The listing builds one solid part. Answer for the finished solid, in the listing's coordinates (mm). Face numbers are marked on the shaded views. A direction names the side the tool comes from. Coordinates: 2 decimals unless noted, no trailing zeros. Order: outer loops, then holes, each group sorted by start corner. A loop starts at its lowest first (then second) coordinate and runs counter-clockwise, first axis right, second up. Notation, with made-up numbers: (26.5, 27) -> (60.5, 27) arc R29 ccw to (60.5, 49) -> close; hole circle Ø10 at (63, 66). An arc over 180 degrees is marked (long way). Return JSON: item names as keys, results as strings.
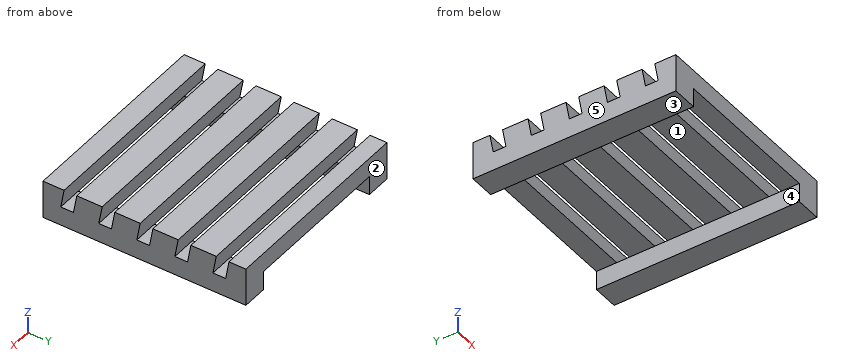
```python
from build123d import *

# Parameters (mm, degrees)
F0_W     = 80
F0_H     = 80
F1_DEPTH = 15
F3_DEPTH = 111
F4_W     = 60
F4_H     = 7.5
F5_DEPTH = 111


with BuildPart() as f1:
    # F0 (on Top) → F1 (new body)
    with BuildSketch(Plane.XY):
        Rectangle(F0_W, F0_H)
    extrude(amount=F1_DEPTH)

    # F2 (on face) → F3 (cut)
    with BuildSketch(Plane.YZ.offset(40)):
        Polygon((-26.677548, 15), (-31.677548, 15), (-33, 7.5), (-28, 7.5), align=None)
        Polygon((-11.677548, 15), (-16.677548, 15), (-18, 7.5), (-13, 7.5), align=None)
        Polygon((3.322452, 15), (-1.677548, 15), (-3, 7.5), (2, 7.5), align=None)
        Polygon((18.322452, 15), (13.322452, 15), (12, 7.5), (17, 7.5), align=None)
        Polygon((32, 7.5), (33.322452, 15), (28.322452, 15), (27, 7.5), align=None)
    extrude(amount=-F3_DEPTH, mode=Mode.SUBTRACT)

    # F4 (on face) → F5 (cut)
    with BuildSketch(Plane.XZ.offset(40)):
        with Locations((0, 3.75)):
            Rectangle(F4_W, F4_H)
    extrude(amount=-F5_DEPTH, mode=Mode.SUBTRACT)


solid = f1.part
```
Item 1: The part is cut by section C-C on y = 35. Determine the outline of the cut face in (x, z).
Answer list:
{"outline": "(-40, 0) -> (-30, 0) -> (-30, 7.5) -> (30, 7.5) -> (30, 0) -> (40, 0) -> (40, 15) -> (-40, 15) -> close"}
Item 2: Which of the six approach directions +Z, -Z, +X, -X, +Y, -Y give full straight-line access (tool end or side, diameter ignored) to the marked faces 1 and 2?
Answer list:
{"face 1": "-Z, +Y, -Y", "face 2": "+Z, -Z, +X, -X, +Y"}
Item 3: The part is cut by section D-D on z = 14. Determine the outline of the cut face in (x, y), plus the area to 3 significant figures.
Answer list:
{"outline": "(-40, -40) -> (40, -40) -> (40, -31.85) -> (-40, -31.85) -> close; (-40, -26.85) -> (40, -26.85) -> (40, -16.85) -> (-40, -16.85) -> close; (-40, -11.85) -> (40, -11.85) -> (40, -1.85) -> (-40, -1.85) -> close; (-40, 3.15) -> (40, 3.15) -> (40, 13.15) -> (-40, 13.15) -> close; (-40, 18.15) -> (40, 18.15) -> (40, 28.15) -> (-40, 28.15) -> close; (-40, 33.15) -> (40, 33.15) -> (40, 40) -> (-40, 40) -> close", "area": "4,400 mm2"}
Item 4: The part is cut by section B-B on z = 1. Determine the outline of the cut face in (x, y), plus the area to 3 significant figures.
Answer list:
{"outline": "(-40, -40) -> (-30, -40) -> (-30, 40) -> (-40, 40) -> close; (30, -40) -> (40, -40) -> (40, 40) -> (30, 40) -> close", "area": "1,600 mm2"}
Item 5: Determine the mould class of the marked faces 3, 4 and 5 for opening direction X: pulls with the +X half, pulls with the -X half, needs draft (parallel to the pull), parting line crosses it, or undercut.
Answer list:
{"face 3": "needs draft", "face 4": "undercut", "face 5": "pulls with the -X half"}
Item 6: Find the intervals of material crossed by probe 1 along X at (y, z) = (-31, 3); probe 2 along Y at (x, z) = (-28.5, 14); probe 3 along Y at (x, z) = (-10.5, 12.5), in increasing order.
Answer list:
{"probe 1": "-40 to -30, 30 to 40", "probe 2": "-40 to -31.85, -26.85 to -16.85, -11.85 to -1.85, 3.15 to 13.15, 18.15 to 28.15, 33.15 to 40", "probe 3": "-40 to -32.12, -27.12 to -17.12, -12.12 to -2.12, 2.88 to 12.88, 17.88 to 27.88, 32.88 to 40"}
Item 7: Flat-ended cylindrical pins translate along their axes: pin 1 (3 mm diameter, centred on x = -18, y = -8.5, fed in from -Z); pin 2 (2.5 mm diameter, centred on x = 33, y = -30, fed in from +Z). Find the tip coordinate at first contact, or state that the pin passes through.
Answer list:
{"pin 1": "z = 7.5", "pin 2": "z = 7.5"}
Item 8: The part is cut by section A-A on x = 7.5. Determine the outline of the cut face in (y, z), plus the area to 4 significant figures.
Answer list:
{"outline": "(-40, 7.5) -> (-33, 7.5) -> (-31.68, 15) -> (-40, 15) -> close; (-28, 7.5) -> (-18, 7.5) -> (-16.68, 15) -> (-26.68, 15) -> close; (-13, 7.5) -> (-3, 7.5) -> (-1.68, 15) -> (-11.68, 15) -> close; (2, 7.5) -> (12, 7.5) -> (13.32, 15) -> (3.32, 15) -> close; (17, 7.5) -> (27, 7.5) -> (28.32, 15) -> (18.32, 15) -> close; (32, 7.5) -> (40, 7.5) -> (40, 15) -> (33.32, 15) -> close", "area": "412.5 mm2"}
